The model under review builds one solid part; all positions refer to its coordinate system, in mm. Give positions to 0.01 mm unless a question says otherwise; leave off trailing zeros. Loops run counter-clockwise (first coordinate to the right, second up) from the corner with the lowest first, then second, coordinate; pieces in that order, holes last. Notation, with made-up numbers: (4.25, 74.25) -> (27.25, 74.25) arc R26 ccw to (27.25, 92.25) -> close; hole circle Ø11 at (34.5, 85.5). An arc over 180 degrees is marked (long way). Write each question's results on one line, items separated by ' | '. Start each with the question number.
Q1. We need section A-A (x = 10.5). Write out the cut boundary in (y, z) (3 decimals).
Q2. We need section B-B (y = 48). Write out the cut boundary in (x, z) (1 decimal).
Q3. Insertion check: pin 1 Ø1.5 at (y, z) = (35, -1) entering from -X; pin 2 Ø1.5 at (x, z) = (34, -1) entering from -Y (3 decimals); pin 3 Ø4.5 at (x, y) = (-106.4, -25.59) entering from -Z. Each pin has a flat end and moves straight along its axis. Give the tip position at first contact, or say it passes through.
Q4. We need section C-C (z = 7.5). Give the number of separate pieces and of enclosed holes in the cut face, plus the area to 3 significant figures.
Q5. Wall thickness on L1, parallel to Y at x = 50.8, z = 5 (3 decimals); L2, parallel to X at y = 23, z = 4.5 (1 decimal); L3, parallel to Y at x = -79, z = 2.5 (3 decimals): over which ranges is each line inside the solid? List them lowest first. Write a range as [from, to].
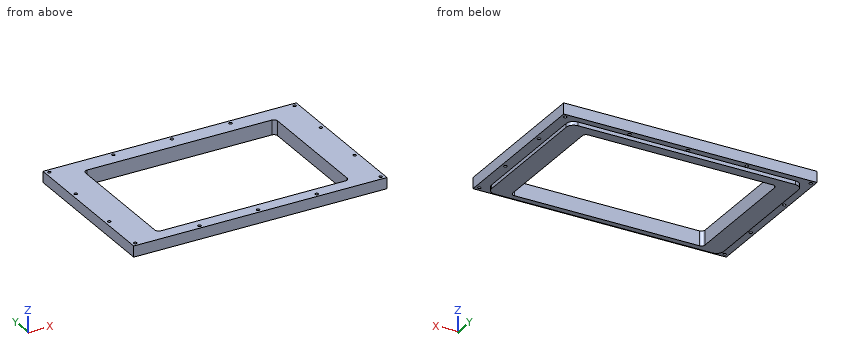
from build123d import *

# Parameters (mm, degrees)
F1_DEPTH = 3.175
F2_W     = 219.71
F2_H     = 137.3124
F3_DEPTH = 9.525
F5_D     = 2.7051


# Not quite as in the source:
# - a feature of the source that left no trace in its solid (it failed there, or was rolled back) is left out


with BuildPart() as f1:
    # F0 (on Top) → F1 (new body)
    with BuildSketch(Plane.XY):
        with BuildLine():
            ThreePointArc((100.71989, 56.515), (98.8600180605, 61.0051280605), (94.36989, 62.865))
            Line((94.36989, 62.865), (-94.36989, 62.865))
            ThreePointArc((-94.36989, 62.865), (-98.8600180605, 61.0051280605), (-100.71989, 56.515))
            Line((-100.71989, 56.515), (-100.71989, -56.515))
            ThreePointArc((-100.71989, -56.515), (-98.8600180605, -61.0051280605), (-94.36989, -62.865))
            Line((-94.36989, -62.865), (94.36989, -62.865))
            ThreePointArc((94.36989, -62.865), (98.8600180605, -61.0051280605), (100.71989, -56.515))
            Line((100.71989, -56.515), (100.71989, 56.515))
        make_face()
        with BuildLine():
            ThreePointArc((83.3755, -54.61), (82.4455640303, -56.8550640303), (80.2005, -57.785))
            Line((80.2005, -57.785), (-80.2005, -57.785))
            ThreePointArc((-80.2005, -57.785), (-82.4455640303, -56.8550640303), (-83.3755, -54.61))
            Line((-83.3755, -54.61), (-83.3755, 50.8))
            ThreePointArc((-83.3755, 50.8), (-82.4455640303, 53.0450640303), (-80.2005, 53.975))
            Line((-80.2005, 53.975), (80.2005, 53.975))
            ThreePointArc((80.2005, 53.975), (82.4455640303, 53.0450640303), (83.3755, 50.8))
            Line((83.3755, 50.8), (83.3755, -54.61))
        make_face(mode=Mode.SUBTRACT)
    extrude(amount=-F1_DEPTH)

    # F2 (on face) → F3 (join)
    with BuildSketch(Plane.XY):
        Rectangle(F2_W, F2_H)
        with BuildLine():
            Line((-80.2005, 53.975), (80.2005, 53.975))
            ThreePointArc((80.2005, 53.975), (82.4455640303, 53.0450640303), (83.3755, 50.8))
            Line((83.3755, 50.8), (83.3755, -54.61))
            ThreePointArc((83.3755, -54.61), (82.4455640303, -56.8550640303), (80.2005, -57.785))
            Line((80.2005, -57.785), (-80.2005, -57.785))
            ThreePointArc((-80.2005, -57.785), (-82.4455640303, -56.8550640303), (-83.3755, -54.61))
            Line((-83.3755, -54.61), (-83.3755, 50.8))
            ThreePointArc((-83.3755, 50.8), (-82.4455640303, 53.0450640303), (-80.2005, 53.975))
        make_face(mode=Mode.SUBTRACT)
    extrude(amount=F3_DEPTH)

    # F5 (through all)
    with Locations(Plane(origin=(0, 0, 0), x_dir=(1, 0, 0), z_dir=(0, 0, -1))):
        with Locations((106.4006, -65.1256), (50.8, -65.1256), (0, -65.1256), (-50.8, -65.1256), (-106.4006, -65.1256), (-106.4006, -25.2095), (-106.4006, 25.5905), (-106.4006, 65.1256), (0, 65.1256), (-50.8, 65.1256), (50.8, 65.1256), (106.4006, 65.1256), (106.4006, 25.5905), (106.4006, -25.2095)):
            Hole(F5_D / 2)


solid = f1.part
Output:
1) outline: (-68.656, 0) -> (-62.865, 0) -> (-62.865, -3.175) -> (-57.785, -3.175) -> (-57.785, 9.525) -> (-68.656, 9.525) -> close; (53.975, -3.175) -> (62.865, -3.175) -> (62.865, 0) -> (68.656, 0) -> (68.656, 9.525) -> (53.975, 9.525) -> close
2) outline: (-109.9, 0) -> (-100.7, 0) -> (-100.7, -3.2) -> (-83.4, -3.2) -> (-83.4, 9.5) -> (-109.9, 9.5) -> close; (83.4, -3.2) -> (100.7, -3.2) -> (100.7, 0) -> (109.9, 0) -> (109.9, 9.5) -> (83.4, 9.5) -> close
3) pin 1: x = -100.72 | pin 2: y = -62.865 | pin 3: z = 0
4) separate pieces: 1 | enclosed holes: 15 | area: 11,500 mm2
5) L1: [-68.656, -66.478], [-63.773, -57.785], [53.975, 63.773], [66.478, 68.656] | L2: [-109.9, -83.4], [83.4, 109.9] | L3: [-68.656, -57.785], [53.975, 68.656]
